Part model, mm, in its own coordinate system. Face numbers are marked on the shaded views. A direction names the side the tool comes from. Round coordinates to 2 decimals unless told otherwise and drop trailing zeros. Write each loop counter-clockwise with the first axis right and the second up, starting at its lowest first coordinate (ties: lowest second). Pieces come first, ordered by that corner, then holes.
```python
from build123d import *

# Parameters (mm, degrees)
SKETCH1_W               = 100
SKETCH1_H               = 90
BOSS_EXTRUDE1_DEPTH     = 6
CUT_EXTRUDE1_REACH      = 69.535
SKETCH2_R               = 12.1
SKETCH3_W               = 10
SKETCH3_H               = 90
BOSS_EXTRUDE2_DEPTH     = 60
SKETCH5_W               = 10
SKETCH5_H               = 10
BOSS_EXTRUDE4_DEPTH     = 60
SKETCH7_R               = 3.5
CUT_EXTRUDE2_DEPTH      = 35
CUT_EXTRUDE3_REACH      = 77.829
SKETCH8_R               = 1.6
CUT_EXTRUDE4_REACH      = 96.239
SKETCH9_R               = 1.6
SKETCH10_R              = 3.5
CUT_EXTRUDE5_DEPTH      = 35
M5_CLEARANCE_HOLE2_D    = 5.5
CUT_EXTRUDE7_REACH      = 127
CUT_EXTRUDE8_DEPTH      = 95.23905772
CUT_EXTRUDE8_DEPTH_BACK = 35
CHAMFER1_SIZE           = 5
CUT_EXTRUDE9_DEPTH      = 35
CUT_EXTRUDE10_REACH     = 127
BOSS_EXTRUDE5_DEPTH     = 10


with BuildPart() as part:
    # Sketch1 → Boss-Extrude1 (new body)
    with BuildSketch(Plane.XY):
        Rectangle(SKETCH1_W, SKETCH1_H)
    extrude(amount=BOSS_EXTRUDE1_DEPTH)

    # Sketch2 → Cut-Extrude1 (cut, up to next)
    with BuildSketch(Plane.XY.offset(6), mode=Mode.PRIVATE) as cut_extrude1_sk1:
        with Locations((-12, -15)):
            Circle(SKETCH2_R)
    cut_extrude1_tool1 = extrude(cut_extrude1_sk1.sketch, amount=-CUT_EXTRUDE1_REACH, mode=Mode.PRIVATE) & part.part
    add(cut_extrude1_tool1.solids().sort_by_distance((-12, -15, 6))[0], mode=Mode.SUBTRACT)

    # Sketch3 → Boss-Extrude2 (add)
    with BuildSketch(Plane(origin=(0, 0, 0), x_dir=(-1, 0, 0), z_dir=(0, 0, -1))):
        with Locations((-45, 0)):
            Rectangle(SKETCH3_W, SKETCH3_H)
    extrude(amount=BOSS_EXTRUDE2_DEPTH)

    # Sketch5 → Boss-Extrude4 (add)
    with BuildSketch(Plane(origin=(0, 0, 0), x_dir=(-1, 0, 0), z_dir=(0, 0, -1))):
        with Locations((40, 40)):
            Rectangle(SKETCH5_W, SKETCH5_H)
    extrude(amount=BOSS_EXTRUDE4_DEPTH)

    # Sketch7 → Cut-Extrude2 (cut)
    with BuildSketch(Plane.XY.offset(6)):
        with Locations((45, 35)):
            Circle(SKETCH7_R)
        with Locations((45, -25)):
            Circle(SKETCH7_R)
    extrude(amount=-CUT_EXTRUDE2_DEPTH, mode=Mode.SUBTRACT)

    # Sketch8 → Cut-Extrude3 (cut, up to next)
    with BuildSketch(Plane.XY.offset(-29), mode=Mode.PRIVATE) as cut_extrude3_sk1:
        with Locations((45, 35)):
            Circle(SKETCH8_R)
    cut_extrude3_tool1 = extrude(cut_extrude3_sk1.sketch, amount=-CUT_EXTRUDE3_REACH, mode=Mode.PRIVATE) & part.part
    # Sketch8 → Cut-Extrude3 (cut, up to next)
    with BuildSketch(Plane.XY.offset(-29), mode=Mode.PRIVATE) as cut_extrude3_sk2:
        with Locations((45, -25)):
            Circle(SKETCH8_R)
    cut_extrude3_tool2 = extrude(cut_extrude3_sk2.sketch, amount=-CUT_EXTRUDE3_REACH, mode=Mode.PRIVATE) & part.part
    add(cut_extrude3_tool1.solids().sort_by_distance((45, 35, -29))[0], mode=Mode.SUBTRACT)
    add(cut_extrude3_tool2.solids().sort_by_distance((45, -25, -29))[0], mode=Mode.SUBTRACT)

    # Sketch9 → Cut-Extrude4 (cut, up to next)
    with BuildSketch(Plane(origin=(0, 0, -60), x_dir=(-1, 0, 0), z_dir=(0, 0, -1)), mode=Mode.PRIVATE) as cut_extrude4_sk1:
        with Locations((40, 40)):
            Circle(SKETCH9_R)
    cut_extrude4_tool1 = extrude(cut_extrude4_sk1.sketch, amount=-CUT_EXTRUDE4_REACH, mode=Mode.PRIVATE) & part.part
    add(cut_extrude4_tool1.solids().sort_by_distance((-40, 40, -60))[0], mode=Mode.SUBTRACT)

    # Sketch10 → Cut-Extrude5 (cut)
    with BuildSketch(Plane.XY.offset(6)):
        with Locations((-40, 40)):
            Circle(SKETCH10_R)
    extrude(amount=-CUT_EXTRUDE5_DEPTH, mode=Mode.SUBTRACT)

    # M5 Clearance Hole2 (through all)
    with Locations(Plane.XY.offset(6)):
        with Locations((-11.992398496, 7.932190932), (-12.437514592, -37.928041631)):
            Hole(M5_CLEARANCE_HOLE2_D / 2)

    # Sketch16 → Cut-Extrude7 (cut, up to next)
    with BuildSketch(Plane(origin=(50, 0, 0), x_dir=(0, 0, -1), z_dir=(1, 0, 0)), mode=Mode.PRIVATE) as cut_extrude7_sk1:
        Polygon((0, 20.599003457), (0, -10.599003457), (21.83860484, 5), align=None)
    cut_extrude7_tool1 = extrude(cut_extrude7_sk1.sketch, amount=-CUT_EXTRUDE7_REACH, mode=Mode.PRIVATE) & part.part
    # Sketch16 → Cut-Extrude7 (cut, up to next)
    with BuildSketch(Plane(origin=(50, 0, 0), x_dir=(0, 0, -1), z_dir=(1, 0, 0)), mode=Mode.PRIVATE) as cut_extrude7_sk2:
        Polygon((54, -10.599003457), (32.16139516, 5), (54, 20.599003457), align=None)
    cut_extrude7_tool2 = extrude(cut_extrude7_sk2.sketch, amount=-CUT_EXTRUDE7_REACH, mode=Mode.PRIVATE) & part.part
    # Sketch16 → Cut-Extrude7 (cut, up to next)
    with BuildSketch(Plane(origin=(50, 0, 0), x_dir=(0, 0, -1), z_dir=(1, 0, 0)), mode=Mode.PRIVATE) as cut_extrude7_sk3:
        Polygon((27, 1.313289171), (5.56139516, -14), (48.43860484, -14), align=None)
    cut_extrude7_tool3 = extrude(cut_extrude7_sk3.sketch, amount=-CUT_EXTRUDE7_REACH, mode=Mode.PRIVATE) & part.part
    # Sketch16 → Cut-Extrude7 (cut, up to next)
    with BuildSketch(Plane(origin=(50, 0, 0), x_dir=(0, 0, -1), z_dir=(1, 0, 0)), mode=Mode.PRIVATE) as cut_extrude7_sk4:
        Polygon((27, 8.686710829), (48.43860484, 24), (5.56139516, 24), align=None)
    cut_extrude7_tool4 = extrude(cut_extrude7_sk4.sketch, amount=-CUT_EXTRUDE7_REACH, mode=Mode.PRIVATE) & part.part
    add(cut_extrude7_tool1.solids().sort_by_distance((50, 5, -7.279535))[0], mode=Mode.SUBTRACT)
    add(cut_extrude7_tool2.solids().sort_by_distance((50, 5, -46.720465))[0], mode=Mode.SUBTRACT)
    add(cut_extrude7_tool3.solids().sort_by_distance((50, -8.89557, -27))[0], mode=Mode.SUBTRACT)
    add(cut_extrude7_tool4.solids().sort_by_distance((50, 18.89557, -27))[0], mode=Mode.SUBTRACT)

    # Sketch17 → Cut-Extrude8 (cut, two sides: drawn at the far end of the back side and taken through both)
    with BuildSketch(Plane.XY.offset(6).offset(-CUT_EXTRUDE8_DEPTH_BACK)):
        Polygon((-114.544785815, 293.179143259), (-50, 35), (-30, -45), (34.544785815, -303.179143259), (-481.813500704, -432.268714889), (-630.903072333, 164.08957163), align=None)
    extrude(amount=CUT_EXTRUDE8_DEPTH + CUT_EXTRUDE8_DEPTH_BACK, mode=Mode.SUBTRACT)

    # Chamfer1
    chamfer1_edges = [part.edges().sort_by_distance(p)[0] for p in [
        (-50, 45, 3),
    ]]
    chamfer(chamfer1_edges, length=CHAMFER1_SIZE)

    # Sketch18 → Cut-Extrude9 (cut)
    with BuildSketch(Plane.XY.offset(6)):
        Polygon((-38.442235936, 30), (-31.851459244, 3.636893232), (-13.002338185, 30), align=None)
        Polygon((-1.606548225, 30), (30.238919993, -1.845468218), (35, -1.845468218), (35, 30), align=None)
    extrude(amount=-CUT_EXTRUDE9_DEPTH, mode=Mode.SUBTRACT)

    # Sketch19 → Cut-Extrude10 (cut, up to next)
    with BuildSketch(Plane(origin=(50, 0, 0), x_dir=(0, 0, -1), z_dir=(1, 0, 0)), mode=Mode.PRIVATE) as cut_extrude10_sk1:
        Polygon((60, -30), (-6, -45), (60, -45), align=None)
    cut_extrude10_tool1 = extrude(cut_extrude10_sk1.sketch, amount=-CUT_EXTRUDE10_REACH, mode=Mode.PRIVATE) & part.part
    add(cut_extrude10_tool1.solids().sort_by_distance((50, -40, -38))[0], mode=Mode.SUBTRACT)

    # Sketch20 → Boss-Extrude5 (add)
    with BuildSketch(Plane(origin=(0, 45, 0), x_dir=(1, 0, 0), z_dir=(0, 1, 0))):
        Polygon((-5, 0), (-35, 60), (-35, 46.583592135), (-11.708203932, 0), align=None)
    extrude(amount=-BOSS_EXTRUDE5_DEPTH)


solid = part.part
```
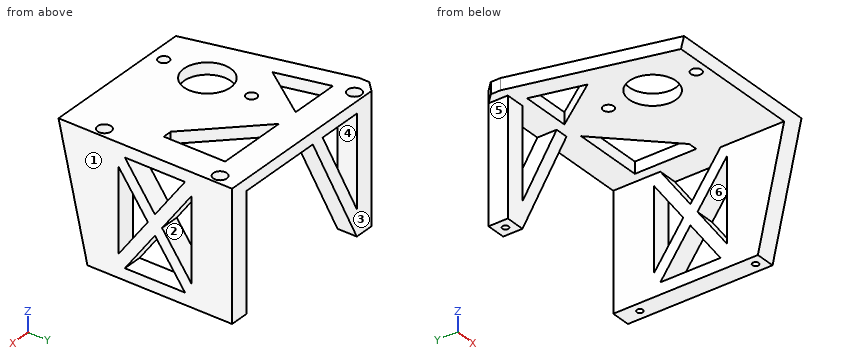
Q1. Mould opens along Y. For the marked faces 1, 2 and 3 say: +Y half, -Y half, draft (parallel to the pull), parting line (faces both ways), or undercut.
Values follow:
face 1: draft
face 2: undercut
face 3: +Y half
Q2. Drop flat-ended pins along their axis: pin 1 (3 mm diameter, centred on y = 24, z = -11, fed in from -X); pin 2 (3 mm diameter, centred on x = 16, z = 1.5, fed in from -Y); pin 3 (4 mm diameter, centred on x = -32.5, z = -39, fed in from +Y); pin 4 (3 mm diameter, centred on x = -29.5, z = 2, fed in from -Y). Give the stop position or say it passes through.
Values follow:
pin 1: stops at x = 40
pin 2: stops at y = -44.32
pin 3: stops at y = 45
pin 4: stops at y = -44.43
Q3. Cut at D-D on y = -18. Write the cut outline in (x, z).
Values follow:
outline: (-36.75, 0) - (-23.72, 0) - (-23.72, 6) - (-36.75, 6) - close; (-0.28, 0) - (40, 0) - (40, -60) - (50, -60) - (50, 6) - (-0.28, 6) - close
Q4. Cut at A-A on z = -35. State how many separate pieces and enclosed holes the cut face has, plus the area to 3 significant figures.
Values follow:
separate pieces: 6
enclosed holes: 3
area: 717 mm2
Q5. Wall check: L1, parallel to Y at x = -11, z = -6.5; L2, parallel to Y at x = 45, z = -41; L3, parallel to Y at x = 45, z = -20. Give the ranges that are in metal, low to high.
Values follow:
L1: y = 35 to 45
L2: y = -34.32 to -26.6, -23.4 to -14, -8.69 to -1.31, 11.31 to 18.69, 24 to 33.4, 36.6 to 45
L3: y = -39.09 to -28.5, -21.5 to -14, -3.69 to 3.69, 6.31 to 13.69, 24 to 31.5, 38.5 to 45
Q6. Which spindle directions (+Z, -Z, +X, -X, +Y, -Y) get a long thin tool onto all of the face, cutting with end or side? Do the marked faces 4, 5 and 6. Say none if no direction does.
Values follow:
face 4: +Y, -Y
face 5: -Z, -X, +Y, -Y
face 6: +X, -X
Q7. Cut at C-C on z = -2. Write the cut outline in (x, y).
Values follow:
outline: (-45, 35) - (-35, 35) - (-35, 45) - (-45, 45) - close; (-12.71, 35) - (-6, 35) - (-6, 45) - (-12.71, 45) - close; (40, -43.18) - (50, -43.18) - (50, -9.17) - (40, -9.17) - close; (40, 19.17) - (50, 19.17) - (50, 45) - (40, 45) - close; hole circle Ø7 at (-40, 40); hole circle Ø7 at (45, -25); hole circle Ø7 at (45, 35)
